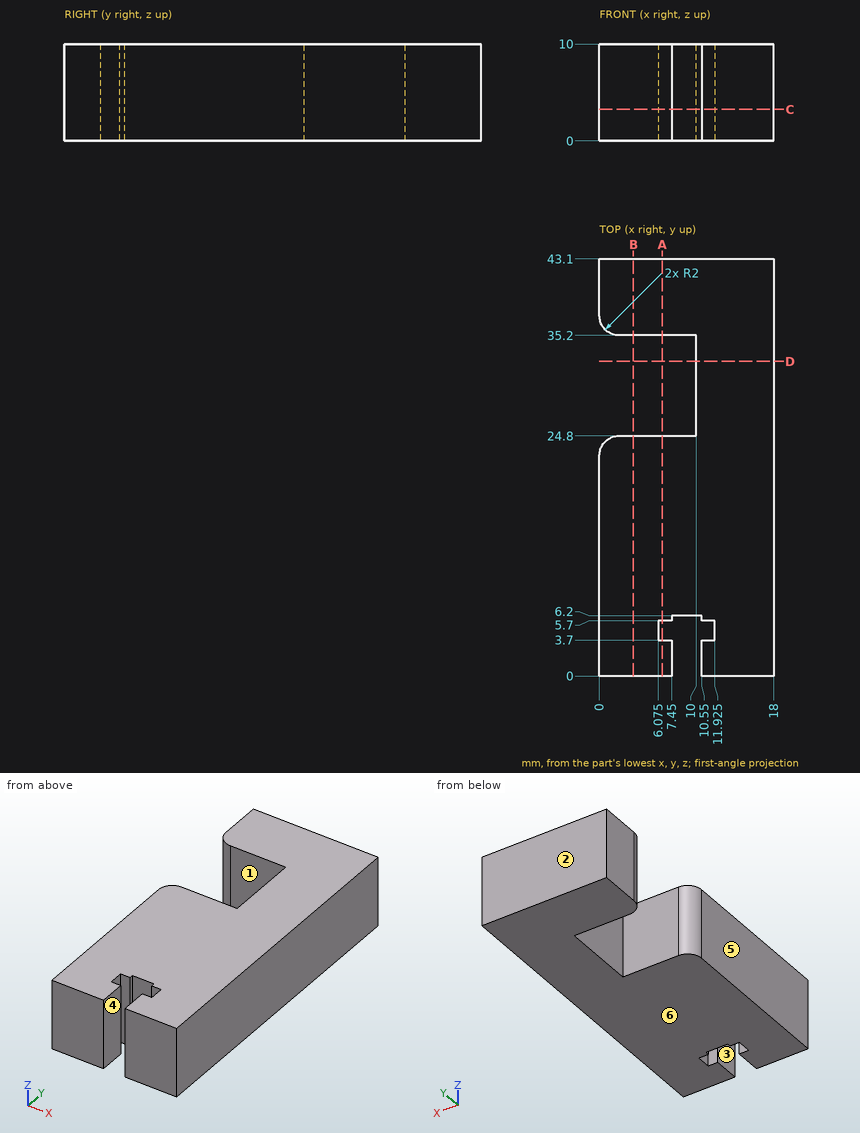
Could you check a few things on this drawing? It's one solid part, dimensions in mm from its lowest x, y, z. A direction names the side the tool comes from. Coordinates: 2 decimals unless noted, no trailing zeros. Loops run counter-clockwise (first coordinate to the right, second up) from the corner with the lowest first, then second, coordinate; pieces in that order, holes last. Notation, with made-up numbers: (4.25, 0) - (24.25, 0) arc R27 ccw to (24.25, 25) - close; hole circle Ø2 at (53.5, 86.5). An arc over 180 degrees is marked (long way). Return JSON: item names as keys, results as strings. Group by question number.
Item 1: If we section it at C-C on z = 3.25: Write out the boundary of the cut face in (x, y) (3 decimals).
Item 2: On a 3-axis mill with a long thin cutter (end or side, diameter ignored), from which of +Z, -Z, +X, -X, +Y, -Y can I reach the whole of each face in a straight line? I mean the marked faces 1, 2 and 3. Say none if no direction works.
Item 3: Will this pin go through, and if not, where does the flat tip stop? P1, Ø5, axis at y = 28.5, z = 6.5, coming from the -X side.
Item 4: If we section it at D-D on y = 32.5: Write out the boundary of the cut face in (x, z).
Item 5: If we section it at B-B on x = 3.5: Write out the boundary of the cut face in (y, z).
Item 6: We'd pull the mould along X, two halves only. Please class the marked faces 4, 5 and 6: +X half, -X half, draft (parallel to the pull), parting line (faces both ways), or undercut.
Item 7: If we section it at A-A on x = 6.5: Write out the boundary of the cut face in (y, z), and give its area (3 significant figures).
Item 8: I need wall thicknesses on line 1 (Y direction, x = 2.25, z = 1); line 2 (Y direction, x = 7.5, z = 2.25); line 3 (X direction, y = 2, z = 3.25). Which ranges of each line are inside material? Lowest first, please. Write a range as from..to.
Calculated:
{
 "1": {"outline": "(0, 0) - (7.45, 0) - (7.45, 3.7) - (6.075, 3.7) - (6.075, 5.7) - (7.45, 5.7) - (7.45, 6.2) - (10.55, 6.2) - (10.55, 5.7) - (11.925, 5.7) - (11.925, 3.7) - (10.55, 3.7) - (10.55, 0) - (18, 0) - (18, 43.1) - (0, 43.1) - (0, 37.2) arc R2 ccw to (2, 35.2) - (10, 35.2) - (10, 24.8) - (2, 24.8) arc R2 ccw to (0, 22.8) - close"},
 "2": {"face 1": "+Z, -Z, -X", "face 2": "+Z, -Z, +X, -X, +Y", "face 3": "+Z, -Z, -Y"},
 "3": {"P1": "stops at x = 10"},
 "4": {"outline": "(10, 0) - (18, 0) - (18, 10) - (10, 10) - close"},
 "5": {"outline": "(0, 0) - (24.8, 0) - (24.8, 10) - (0, 10) - close; (35.2, 0) - (43.1, 0) - (43.1, 10) - (35.2, 10) - close"},
 "6": {"face 4": "undercut", "face 5": "-X half", "face 6": "draft"},
 "7": {"outline": "(0, 0) - (3.7, 0) - (3.7, 10) - (0, 10) - close; (5.7, 0) - (24.8, 0) - (24.8, 10) - (5.7, 10) - close; (35.2, 0) - (43.1, 0) - (43.1, 10) - (35.2, 10) - close", "area": "307 mm^2"},
 "8": {"line 1": "y = 0..24.8, 35.2..43.1", "line 2": "y = 6.2..24.8, 35.2..43.1", "line 3": "x = 0..7.45, 10.55..18"}
}
